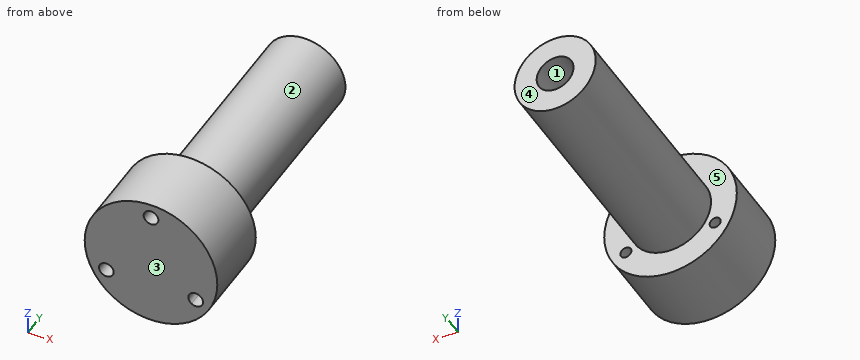
```python
from build123d import *

# Parameters (mm, degrees)
F0_R     = 9
F1_DEPTH = 20
F2_R     = 0.75
F3_DEPTH = 8
F4_R     = 9
F4_R_2   = 5.5
F5_DEPTH = 30
F6_DEPTH = 10
F7_R     = 2.5
F8_DEPTH = 10


with BuildPart() as f1:
    # F0 (on Front) → F1 (new body, symmetric)
    with BuildSketch(Plane.XZ):
        Circle(F0_R)
    extrude(amount=F1_DEPTH, both=True)

    # F2 (on face) → F3 (cut)
    with BuildSketch(Plane.XZ.offset(20)):
        with BuildLine():
            ThreePointArc((1, 7), (-0.035737, 7.999361), (-0.997446, 6.928571))
            ThreePointArc((-0.997446, 6.928571), (0, 6), (0.997446, 6.928571))
            ThreePointArc((0.997446, 6.928571), (0.999361, 6.964263), (1, 7))
        make_face()
        with Locations((0, 7)):
            Circle(F2_R, mode=Mode.SUBTRACT)
        with BuildLine():
            ThreePointArc((-5.062178, -3.5), (-5.531548, -2.652396), (-6.499042, -2.600472))
            ThreePointArc((-6.499042, -2.600472), (-6.928203, -4), (-5.501596, -4.328099))
            ThreePointArc((-5.501596, -4.328099), (-5.178837, -3.968731), (-5.062178, -3.5))
        make_face()
        with Locations((-6.062178, -3.5)):
            Circle(F2_R, mode=Mode.SUBTRACT)
        with BuildLine():
            ThreePointArc((7.062178, -3.5), (6.909781, -2.96937), (6.499042, -2.600472))
            ThreePointArc((6.499042, -2.600472), (5.196152, -3), (5.501596, -4.328099))
            ThreePointArc((5.501596, -4.328099), (6.530909, -4.383341), (7.062178, -3.5))
        make_face()
        with Locations((6.062178, -3.5)):
            Circle(F2_R, mode=Mode.SUBTRACT)
    extrude(amount=-F3_DEPTH, mode=Mode.SUBTRACT)

    # F4 (on face) → F5 (cut)
    with BuildSketch(Plane(origin=(0, 20, 0), x_dir=(-1, 0, 0), z_dir=(0, 1, 0))):
        Circle(F4_R)
        Circle(F4_R_2, mode=Mode.SUBTRACT)
    extrude(amount=-F5_DEPTH, mode=Mode.SUBTRACT)

    # F2 (on face) → F6 (cut)
    with BuildSketch(Plane.XZ.offset(20)):
        with Locations((-6.062178, -3.5)):
            Circle(F2_R)
        with Locations((0, 7)):
            Circle(F2_R)
        with Locations((6.062178, -3.5)):
            Circle(F2_R)
    extrude(amount=-F6_DEPTH, mode=Mode.SUBTRACT)

    # F7 (on face) → F8 (cut)
    with BuildSketch(Plane(origin=(0, 20, 0), x_dir=(-1, 0, 0), z_dir=(0, 1, 0))):
        Circle(F7_R)
    extrude(amount=-F8_DEPTH, mode=Mode.SUBTRACT)


solid = f1.part
```
Could you check a few things on this model? Use its own coordinates, in mm. Face numbers are marked on the shaded views. A direction names the side the tool comes from. Coordinates: 2 decimals unless noted, no trailing zeros. Loops run counter-clockwise (first coordinate to the right, second up) from the corner with the lowest first, then second, coordinate; pieces in that order, holes last. Notation, with made-up numbers: M -18,30.5 L 32,30.5 A8 ccw 32,39.5 Z; hole C -1.5,60.25 d11. An arc over 180 degrees is marked long. Put each result on its own line as item: value. Start each with the question number.
(1) Suppose I cut it at B-B on z = 0. Please give me the cut outline in (x, y), then the cut area to 3 significant figures.
(2) Suppose I cut it at D-D on y = -9.5. Please give me the cut outline in (x, z), then the cut area to 3 significant figures.
(3) Will these pins go through, and if not, where does the flat tip stop? P1, Ø4, axis at y = 16, z = -4.5, coming from the -X side; P2, Ø1.7, axis at x = 6.06, z = -3.5, coming from the -Y side; P3, Ø2.5, axis at x = 1, z = 0.5, coming from the +Y side; P4, Ø1.4, axis at x = -6.06, z = -3.5, coming from the -Y side (3 decimals).
(4) I need wall thicknesses on line 1 (Z direction, x = 0, y = -11.4); line 2 (Z direction, x = 0, y = -13); line 3 (Y direction, x = 2.5, z = -5.5). Which ranges of each line are inside material? Lowest first, please. Write a range as from..to.
(5) Suppose I cut it at C-C on x = 2. Please give me the cut outline in (y, z).
(6) For the marked faces 4 and 5, which set-ups out of +Z, -Z, +X, -X, +Y, -Y let a thin tool reach every point of the face, with its end or its side?
(7) Thinking about a two-plate mould opening in X: for the marked faces 1, 2 and 3, which applies, pulls with the +X half, pulls with the -X half, needs draft (parallel to the pull), parting line crosses it, or undercut?
(8) Suppose I cut it at A-A on x = 0. Please give me the cut outline in (y, z).
Solutions:
1. outline: M -9,-20 L 9,-20 L 9,-10 L 5.5,-10 L 5.5,20 L 2.5,20 L 2.5,10 L -2.5,10 L -2.5,20 L -5.5,20 L -5.5,-10 L -9,-10 Z
1. area: 460 mm2
2. outline: C 0,0 d11
2. area: 95.0 mm2
3. P1: stops at x = -4.9
3. P2: stops at y = -12
3. P3: stops at y = 10
3. P4: passes through
4. line 1: z = -9..6.25, 7.75..9
4. line 2: z = -9..6, 8..9
4. line 3: y = -20..-10
5. outline: M -20,-8.77 L -10,-8.77 L -10,-5.12 L 20,-5.12 L 20,-1.5 L 10,-1.5 L 10,1.5 L 20,1.5 L 20,5.12 L -10,5.12 L -10,8.77 L -20,8.77 Z
6. face 4: +Z, -Z, +X, -X, +Y
6. face 5: +Y
7. face 1: undercut
7. face 2: parting line crosses it
7. face 3: needs draft
8. outline: M -20,-9 L -10,-9 L -10,-5.5 L 20,-5.5 L 20,-2.5 L 10,-2.5 L 10,2.5 L 20,2.5 L 20,5.5 L -10,5.5 L -10,6.25 L -12,6.25 L -12,6 L -20,6 Z; M -20,8 L -12,8 L -12,7.75 L -10,7.75 L -10,9 L -20,9 Z
